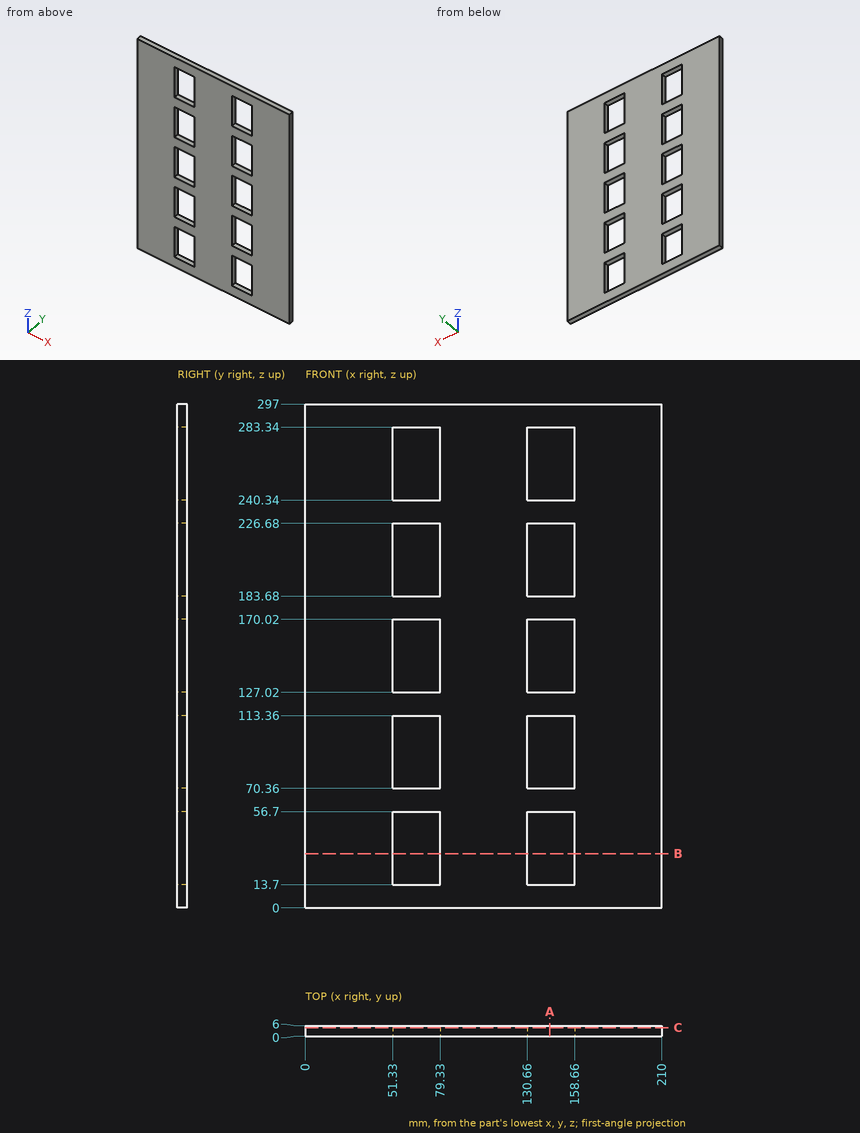
Can you work these out from the drawing? Everything is in mm from the part's minimum corner. Give positions to 0.01 mm unless a question says otherwise; leave off trailing zeros. Order: outer loops, then holes, each group sorted by start corner. A loop starts at its lowest first (then second) coordinate and runs counter-clockwise, first axis right, second up. Notation, with made-up numbers: M -2,42 L 11,42 A9 ccw 11,54 Z; hole C -12.75,12.25 d7. An arc over 180 degrees is marked long. Write item = value, one per line. Start each with the question number.
Q1. Suppose I cut it at C-C (y = 5). Count the separate pieces of the cut face and the enclosed holes in it, plus the area to 3 significant figures.
Q2. Suppose I cut it at A-A (x = 144). Write out the boundary of the cut face in (y, z).
Q3. I need wall thicknesses on probe 1 along X at (y, z) = (5.6, 275); probe 2 along Z at (x, y) = (158.5, 3.05). Which ranges of each line are inside material? Lowest first, please. Write a range as [from, to].
Q4. Suppose I cut it at B-B (z = 32). Write out the boundary of the cut face in (x, y), plus the area to 3 significant figures.
Check result:
q1.separate_pieces = 1
q1.enclosed_holes = 10
q1.area = 50,300 mm2
q2.outline = M 0,0 L 6,0 L 6,13.7 L 0,13.7 Z; M 0,56.7 L 6,56.7 L 6,70.36 L 0,70.36 Z; M 0,113.36 L 6,113.36 L 6,127.02 L 0,127.02 Z; M 0,170.02 L 6,170.02 L 6,183.68 L 0,183.68 Z; M 0,226.68 L 6,226.68 L 6,240.34 L 0,240.34 Z; M 0,283.34 L 6,283.34 L 6,297 L 0,297 Z
q3.probe_1 = [0, 51.33], [79.33, 130.66], [158.66, 210]
q3.probe_2 = [0, 13.7], [56.7, 70.36], [113.36, 127.02], [170.02, 183.68], [226.68, 240.34], [283.34, 297]
q4.outline = M 0,0 L 51.33,0 L 51.33,6 L 0,6 Z; M 79.33,0 L 130.66,0 L 130.66,6 L 79.33,6 Z; M 158.66,0 L 210,0 L 210,6 L 158.66,6 Z
q4.area = 924 mm2
